```python
from build123d import *

# Parameters (mm, degrees)
F0_W     = 187.325
F0_H     = 40.64
F0_W_2   = 19.304
F0_H_2   = 36.83
F1_DEPTH = 3.175
F2_R     = 1.524
F3_DEPTH = 6.35


with BuildPart() as f1:
    # F0 (on Top) → F1 (new body)
    with BuildSketch(Plane.XY):
        with Locations((50.084582, -2.391732)):
            Rectangle(F0_W, F0_H)
        with Locations((50.148082, -2.391732)):
            Rectangle(F0_W_2, F0_H_2, mode=Mode.SUBTRACT)
        with Locations((-23.765918, -2.391732)):
            Rectangle(F0_W_2, F0_H_2, mode=Mode.SUBTRACT)
        with Locations((13.191082, -2.391732)):
            Rectangle(F0_W_2, F0_H_2, mode=Mode.SUBTRACT)
        with Locations((87.105082, -2.391732)):
            Rectangle(F0_W_2, F0_H_2, mode=Mode.SUBTRACT)
        with Locations((123.935082, -2.391732)):
            Rectangle(F0_W_2, F0_H_2, mode=Mode.SUBTRACT)
    extrude(amount=F1_DEPTH)

    # F2 (on face) → F3 (cut, symmetric)
    with BuildSketch(Plane.XY.offset(3.175)):
        with Locations((-14.113918, -2.391732)):
            Circle(F2_R)
        with Locations((22.843082, -2.391732)):
            Circle(F2_R)
        with Locations((59.800082, -2.391732)):
            Circle(F2_R)
        with Locations((96.757082, -2.391732)):
            Circle(F2_R)
        with Locations((133.587082, -2.391732)):
            Circle(F2_R)
    extrude(amount=F3_DEPTH, both=True, mode=Mode.SUBTRACT)


solid = f1.part
```
Check sheet for the modelled part. Datum: model origin and axes. Units: mm. Give positions to 0.01 mm unless a question says otherwise; leave off trailing zeros. Loops run counter-clockwise (first coordinate to the right, second up) from the corner with the lowest first, then second, coordinate; pieces in that order, holes last. Notation, with made-up numbers: (28, 49.5) - (34, 49.5) arc R20 cw to (34, 71.5) - close; hole circle Ø1 at (50.5, -6). An arc over 180 degrees is marked (long way). One line per question, with ' | ' between items. Start each with the question number.
1. Cross-section at C-C, the plane x = 11.5. Enter the section's corners in (y, z) (3 decimals), plus the area to 3 significant figures.
2. Cross-section at B-B, the plane y = 14. Enter the section's corners in (x, z) (3 decimals).
3. Draft check along Y on faces 1 (the flat face through (28, -2, 0)), 2 (the flat face through (49, -22.712, 2)), 3 (the flat face through (-24, -20.807, 2)). Enter one of: released by +Y, released by -Y, zero draft, split by the parting line, or undercut.
4. Cross-section at A-A, the plane z = 1.5. Give the number of separate pieces and of enclosed holes in the cut face, plus the area to 3 significant figures.
5. Gauge pin test, flat end, axial feed: pin 1 Ø3 at (x, y) = (28.5, -9.5) entering from -Z. Record the tip position at first contact, or that the pin passes through.
6. Material ranges on line 1 along X through (y, z) = (14, 2.8); line 2 along Y through (x, z) = (89.5, 1.7); line 3 along X through (y, z) = (-3, 1), recorded low to high. Write a range as [from, to].
Check result:
1) outline: (-22.712, 0) - (-20.807, 0) - (-20.807, 3.175) - (-22.712, 3.175) - close; (16.023, 0) - (17.928, 0) - (17.928, 3.175) - (16.023, 3.175) - close | area: 12.1 mm2
2) outline: (-43.578, 0) - (-33.418, 0) - (-33.418, 3.175) - (-43.578, 3.175) - close; (-14.114, 0) - (3.539, 0) - (3.539, 3.175) - (-14.114, 3.175) - close; (22.843, 0) - (40.496, 0) - (40.496, 3.175) - (22.843, 3.175) - close; (59.8, 0) - (77.453, 0) - (77.453, 3.175) - (59.8, 3.175) - close; (96.757, 0) - (114.283, 0) - (114.283, 3.175) - (96.757, 3.175) - close; (133.587, 0) - (143.747, 0) - (143.747, 3.175) - (133.587, 3.175) - close
3) face 1: zero draft | face 2: released by -Y | face 3: undercut
4) separate pieces: 1 | enclosed holes: 5 | area: 4,040 mm2
5) pin 1: stops at z = 0
6) line 1: x = [-43.58, -33.42], [-14.11, 3.54], [22.84, 40.5], [59.8, 77.45], [96.76, 114.28], [133.59, 143.75] | line 2: y = [-22.71, -20.81], [16.02, 17.93] | line 3: x = [-43.58, -33.42], [-12.72, 3.54], [24.24, 40.5], [61.2, 77.45], [98.15, 114.28], [134.98, 143.75]
